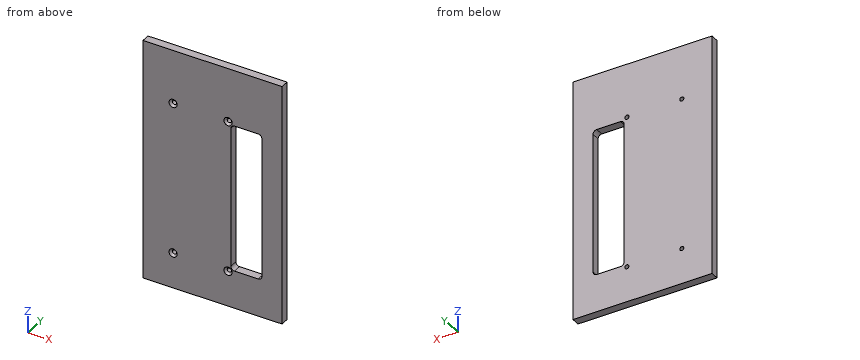
```python
from build123d import *

# Parameters (mm, degrees)
SKETCH1_W           = 152
SKETCH1_H           = 262
BOSS_EXTRUDE1_DEPTH = 9
SKETCH2_R           = 2.25
CUT_EXTRUDE1_DEPTH  = 181.917108091


with BuildPart() as part:
    # Sketch1 → Boss-Extrude1 (new body)
    with BuildSketch(Plane(origin=(0, 0, 0), x_dir=(1, 0, 0), z_dir=(0, 1, 0))):
        with Locations((-37, -10)):
            Rectangle(SKETCH1_W, SKETCH1_H)
        with BuildLine():
            Line((13, 80), (-13, 80))
            ThreePointArc((-13, 80), (-15.828427125, 78.828427125), (-17, 76))
            Line((-17, 76), (-17, -76))
            ThreePointArc((-17, -76), (-15.828427125, -78.828427125), (-13, -80))
            Line((-13, -80), (13, -80))
            ThreePointArc((13, -80), (15.828427125, -78.828427125), (17, -76))
            Line((17, -76), (17, 76))
            ThreePointArc((17, 76), (15.828427125, 78.828427125), (13, 80))
        make_face(mode=Mode.SUBTRACT)
    extrude(amount=BOSS_EXTRUDE1_DEPTH)

    # Sketch2 → Cut-Extrude1 (cut, through all)
    with BuildSketch(Plane.XZ):
        with Locations(Location((-20, 82.5, 0), (0, 0, 270))):
            Circle(SKETCH2_R)
        with Locations(Location((-80, 82.5, 0), (0, 0, 270))):
            Circle(SKETCH2_R)
        with Locations(Location((-20, -82.5, 0), (0, 0, 270))):
            Circle(SKETCH2_R)
        with Locations(Location((-80, -82.5, 0), (0, 0, 270))):
            Circle(SKETCH2_R)
    extrude(amount=-CUT_EXTRUDE1_DEPTH, mode=Mode.SUBTRACT)

    # Cut-Extrude2 cone 1 section (through the dimple's axis) → Cut-Extrude2 (revolve, cut)
    with BuildSketch(Plane(origin=(-80, 0, 82.5), x_dir=(0, 0, -1), z_dir=(1, 0, 0))):
        Polygon((0, 0), (4.5, 0), (0, 4.5), align=None)
    revolve(axis=Axis((-80, 0, 82.5), (0, 1, 0)), mode=Mode.SUBTRACT)

    # Cut-Extrude2 cone 2 section (through the dimple's axis) → Cut-Extrude2 cone 2 (revolve, cut)
    with BuildSketch(Plane(origin=(-20, 0, 82.5), x_dir=(0, 0, -1), z_dir=(1, 0, 0))):
        Polygon((0, 0), (4.5, 0), (0, 4.5), align=None)
    revolve(axis=Axis((-20, 0, 82.5), (0, 1, 0)), mode=Mode.SUBTRACT)

    # Cut-Extrude2 cone 3 section (through the dimple's axis) → Cut-Extrude2 cone 3 (revolve, cut)
    with BuildSketch(Plane(origin=(-20, 0, -82.5), x_dir=(0, 0, -1), z_dir=(1, 0, 0))):
        Polygon((0, 0), (4.5, 0), (0, 4.5), align=None)
    revolve(axis=Axis((-20, 0, -82.5), (0, 1, 0)), mode=Mode.SUBTRACT)

    # Cut-Extrude2 cone 4 section (through the dimple's axis) → Cut-Extrude2 cone 4 (revolve, cut)
    with BuildSketch(Plane(origin=(-80, 0, -82.5), x_dir=(0, 0, -1), z_dir=(1, 0, 0))):
        Polygon((0, 0), (4.5, 0), (0, 4.5), align=None)
    revolve(axis=Axis((-80, 0, -82.5), (0, 1, 0)), mode=Mode.SUBTRACT)


solid = part.part
```
Input: part model. Units: mm. Frame: model coordinates. Round coordinates to 2 decimals unless told otherwise and drop trailing zeros. Write each loop counter-clockwise with the first axis right and the second up, starting at its lowest first coordinate (ties: lowest second). Pieces come first, ordered by that corner, then holes. Notation, with made-up numbers: M 33,7.5 L 79,7.5 A19 cw 79,25.5 Z; hole C -2,56.25 d11. An arc over 180 degrees is marked long. Write each question's results on one line, items separated by ' | '.
Q1. Section query A-A (z = -30). Return loops of the section in (x, y).
Results:
outline: M -113,0 L -17,0 L -17,9 L -113,9 Z; M 17,0 L 39,0 L 39,9 L 17,9 Z
Q2. Line query: line 1 along X through (y, z) = (4.75, -82.5); line 2 along Z through (x, y) = (13, 7); line 3 along Z through (x, y) = (-81.5, 3.5). Output: solid intervals per line, ascending.
Results:
line 1: x = -113 to -82.25, -77.75 to -22.25, -17.75 to 39 | line 2: z = -121 to -80, 80 to 141 | line 3: z = -121 to -84.18, -80.82 to 80.82, 84.18 to 141
Q3. Section query B-B (y = 4). Return loops of the section in (x, z), and give its area (3 significant figures).
Results:
outline: M -113,-121 L 39,-121 L 39,141 L -113,141 Z; hole C -80,-82.5 d4.5; hole C -80,82.5 d4.5; hole C -20,-82.5 d4.5; hole C -20,82.5 d4.5; hole M -17,-76 A4 ccw -13,-80 L 13,-80 A4 ccw 17,-76 L 17,76 A4 ccw 13,80 L -13,80 A4 ccw -17,76 Z | area: 34,300 mm^2
Q4. Pin query (flat end, axial travel): P1, Ø6, axis at x = -20, z = -82.5, coming from the +Y side; P2, Ø6, axis at x = -80, z = 82.5, coming from the -Y side. Return the tip coordinate at first contact, or that it passes through.
Results:
P1: stops at y = 9 | P2: stops at y = 1.5
